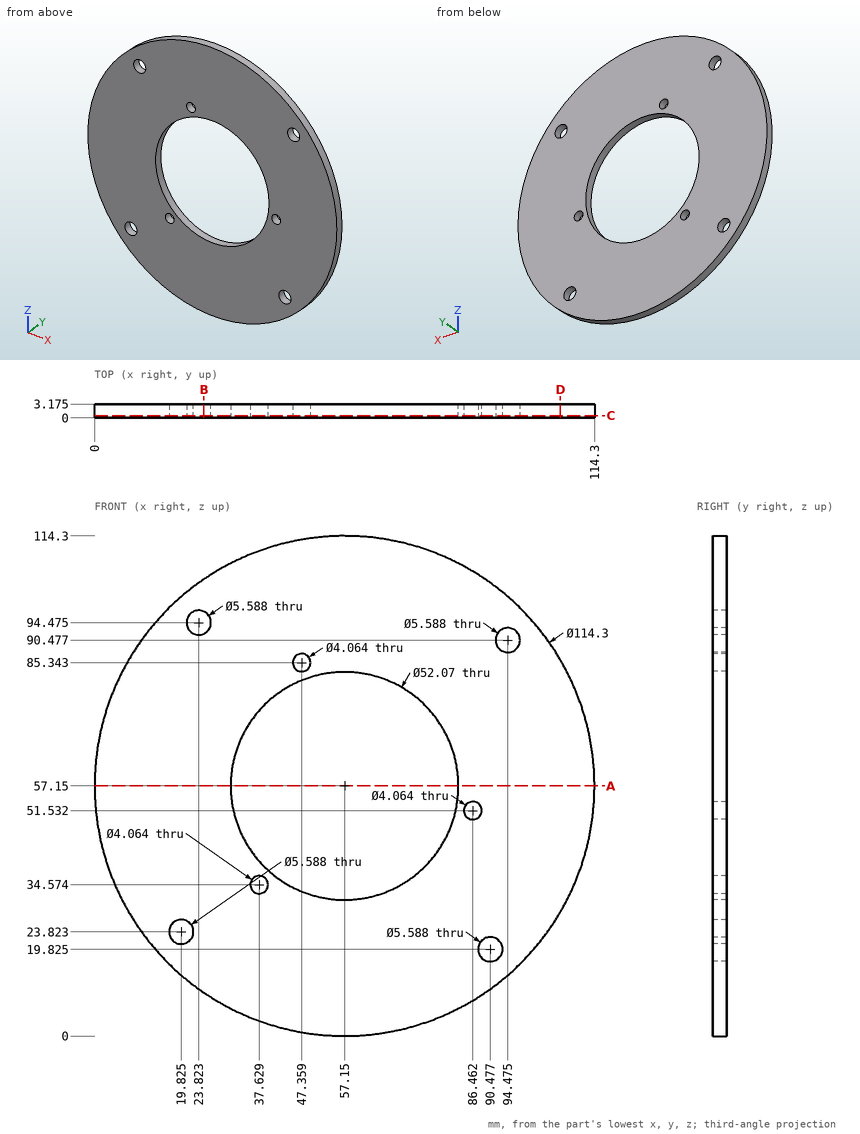
Could you check a few things on this drawing? It's one solid part, dimensions in mm from its lowest x, y, z. Coordinates: 2 decimals unless noted, no trailing zeros. Loops run counter-clockwise (first coordinate to the right, second up) from the corner with the lowest first, then second, coordinate; pieces in that order, holes last. Notation, with made-up numbers: (-19.75, 35.25) - (25.25, 35.25) arc R34 cw to (25.25, 67.25) - close; hole circle Ø3 at (4, 82.5). An arc over 180 degrees is marked (long way). Answer as a JSON object with one key per item and string values. Group by question number.
Item 1: If we section it at D-D (x = 106.5): List the corners of the cut face in (y, z) for me (1 decimal).
Item 2: If we section it at C-C (y = 0.5): State how many separate pieces and enclosed holes the cut face has.
Item 3: If we section it at B-B (x = 25): List the corners of the cut face in (y, z) for me (1 decimal), plus the area to 3 significant figures.
Item 4: For pin 1 (3.5 mm diameter, centred on x = 94.47, z = 90.48, fed in from -Y), with a flat end and sliding along its axis, tell me the tip position at first contact or that it passes through.
Item 5: If I drill on L1, parallel to X at y = 1.1, z = 56; L2, parallel to Z at x = 57.15, y = 2.4 (1 decimal); L3, parallel to X at y = 2.6, z = 52 (1 decimal), over which ranges is the centre line in solid material (lowest first)? Write a range as from..to.
Item 6: If we section it at A-A (z = 57.15): List the corners of the cut face in (x, y) for me (1 decimal).
Returned:
{
 "1": {"outline": "(0, 28.3) - (3.2, 28.3) - (3.2, 86) - (0, 86) - close"},
 "2": {"separate pieces": "1", "enclosed holes": "8"},
 "3": {"outline": "(0, 9.9) - (3.2, 9.9) - (3.2, 91.9) - (0, 91.9) - close; (0, 97) - (3.2, 97) - (3.2, 104.4) - (0, 104.4) - close", "area": "284 mm²"},
 "4": {"pin 1": "passes through"},
 "5": {"L1": "x = 0.01..31.14, 83.16..114.29", "L2": "z = 0..31.1, 83.2..114.3", "L3": "x = 0.2..31.6, 82.7..84.5, 88.4..114.1"},
 "6": {"outline": "(0, 0) - (31.1, 0) - (31.1, 3.2) - (0, 3.2) - close; (83.2, 0) - (114.3, 0) - (114.3, 3.2) - (83.2, 3.2) - close"}
}
